Geometry check sheet. Reference: the model listing, model coordinates, mm. Face numbers are marked on the shaded views. A direction names the side the tool comes from. Give positions to 0.01 mm unless a question says otherwise; leave off trailing zeros. Order: outer loops, then holes, each group sorted by start corner. A loop starts at its lowest first (then second) coordinate and runs counter-clockwise, first axis right, second up.
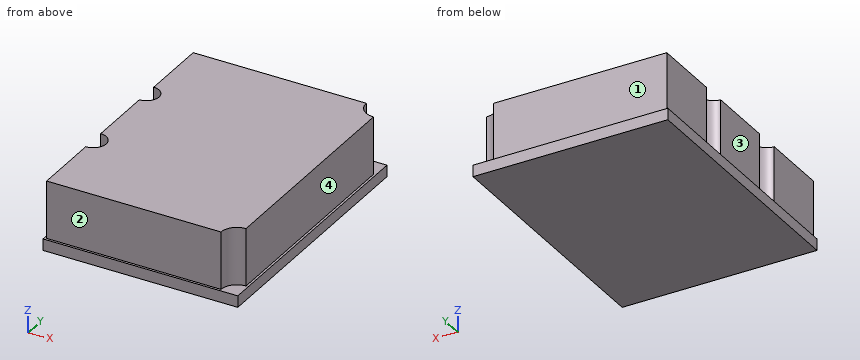
from build123d import *

# Parameters (mm, degrees)
F0_W     = 165
F0_H     = 220
F1_DEPTH = 50
F3_DEPTH = 50
F4_R     = 10.776099
F4_R_2   = 11.209408
F5_DEPTH = 50
F7_DEPTH = 10


with BuildPart() as f1:
    # F0 (on Top) → F1 (new body)
    with BuildSketch(Plane.XY):
        with Locations((-98.687344, -15.532274)):
            Rectangle(F0_W, F0_H)
    extrude(amount=F1_DEPTH)

    # F2 (on face) → F3 (cut)
    with BuildSketch(Plane.XY.offset(50)):
        with BuildLine():
            Line((-16.187344, -125.532274), (-16.187344, -111.789186))
            ThreePointArc((-16.187344, -111.789186), (-25.905174, -115.814443), (-29.930431, -125.532274))
            Line((-29.930431, -125.532274), (-16.187344, -125.532274))
        make_face()
        with BuildLine():
            Line((-16.187344, 94.467726), (-31.029011, 94.467726))
            ThreePointArc((-31.029011, 94.467726), (-26.681987, 83.973083), (-16.187344, 79.626059))
            Line((-16.187344, 79.626059), (-16.187344, 94.467726))
        make_face()
        with BuildLine():
            ThreePointArc((-2.444256, -125.532274), (-6.469513, -115.814443), (-16.187344, -111.789186))
            Line((-16.187344, -111.789186), (-16.187344, -125.532274))
            Line((-16.187344, -125.532274), (-29.930431, -125.532274))
            ThreePointArc((-29.930431, -125.532274), (-16.187344, -139.275361), (-2.444256, -125.532274))
        make_face()
        with BuildLine():
            ThreePointArc((-16.187344, 79.626059), (-5.6927, 83.973083), (-1.345676, 94.467726))
            ThreePointArc((-1.345676, 94.467726), (-16.187344, 109.309394), (-31.029011, 94.467726))
            Line((-31.029011, 94.467726), (-16.187344, 94.467726))
            Line((-16.187344, 94.467726), (-16.187344, 79.626059))
        make_face()
    extrude(amount=-F3_DEPTH, mode=Mode.SUBTRACT)

    # F4 (on face) → F5 (cut)
    with BuildSketch(Plane.XY.offset(50)):
        with Locations((-181.187344, 24.467726)):
            Circle(F4_R)
        with Locations((-181.187344, -55.532274)):
            Circle(F4_R_2)
    extrude(amount=-F5_DEPTH, mode=Mode.SUBTRACT)

    # F6 (on face) → F7 (join)
    with BuildSketch(Plane(origin=(0, 0, 0), x_dir=(1, 0, 0), z_dir=(0, 0, -1))):
        Polygon((-14.187344, 127.532274), (-181.187344, 127.532274), (-183.187344, 127.532274), (-183.187344, 125.532274), (-183.187344, -96.467726), (-159.191355, -96.467726), (-14.187344, -96.467726), (-14.187344, -65.397188), align=None)
    extrude(amount=F7_DEPTH)


solid = f1.part
Item 1: Sectioned sample at B-B (y = -94). Enter the section's corners in (x, z), and give its area (3 significant figures).
Reported:
outline: (-183.19, -10) - (-14.19, -10) - (-14.19, 0) - (-16.19, 0) - (-16.19, 50) - (-181.19, 50) - (-181.19, 0) - (-183.19, 0) - close
area: 9,940 mm2
Item 2: Scan lines: L1, parallel to X at y = 6.5, z = 21; L2, parallel to Y at x = -62, z = 19; L3, parallel to Z at x = -173, y = -52. Record each from-to range of solid material in increasing order.
Reported:
L1: x = -181.19 to -16.19
L2: y = -125.53 to 94.47
L3: z = -10 to 0
Item 3: Gauge pin test, flat ends, axial feed: pin 1 (12 mm diameter, centred on y = -62, z = 16, fed in from +X); pin 2 (2 mm diameter, centred on y = -102, z = 36, fed in from -X); pin 3 (1 mm diameter, centred on x = -148, z = 42, fed in from +Y). Record the tip position at first contact, or that the pin passes through.
Reported:
pin 1: stops at x = -16.19
pin 2: stops at x = -181.19
pin 3: stops at y = 94.47
Item 4: Set-up check for the marked faces 1, 2, 3 and 4: record each of +Z, -Z, +X, -X, +Y, -Y from which the full face is reachable in a straight line by a thin tool's end or side.
Reported:
face 1: +Z, +X, -X, +Y
face 2: +Z, +X, -X, -Y
face 3: +Z, -X, +Y, -Y
face 4: +Z, +X, +Y, -Y
Item 5: Sectioned sample at A-A (z = 13). Enter the section's corners in (x, y), and give its area (3 significant figures).
Reported:
outline: (-181.19, -125.53) - (-29.93, -125.53) arc R13.74 cw to (-16.19, -111.79) - (-16.19, 79.63) arc R14.84 cw to (-31.03, 94.47) - (-181.19, 94.47) - (-181.19, 35.24) arc R10.78 cw to (-181.19, 13.69) - (-181.19, -44.32) arc R11.21 cw to (-181.19, -66.74) - close
area: 35,600 mm2
